Geometry: see drawing. Coordinates: mm, zero at the bounding-box minimum. Round coordinates to 2 decimals unless told otherwise and drop trailing zeros. Write each loop counter-clockwise with the first axis right and the second up, starting at its lowest first coordinate (ties: lowest second). Pieces come first, ordered by that corner, then holes. Notation, with made-up numbers: (-29, 24.25) - (28, 24.25) arc R18 cw to (28, 59.25) - close; hole circle Ø11 at (6.25, 38.25). An arc over 180 degrees is marked (long way). One line per item, written item: value. Start each with the question number.
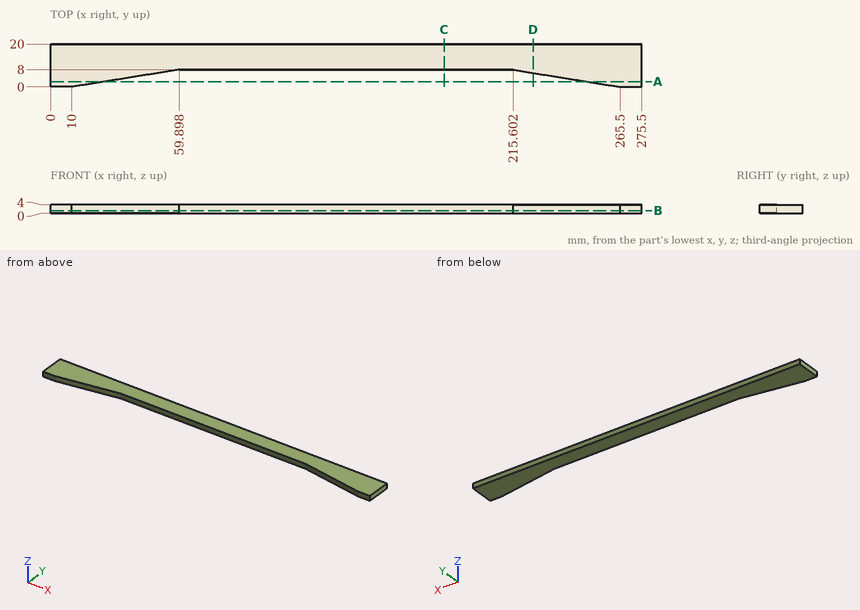
Q1. Cut plane B-B, the plane z = 1.35. Output: boundary loops of the cut face in (x, y), and give its area (4 significant figures).
Q2. Cut plane C-C, the plane x = 183.5. Output: boundary loops of the cut face in (y, z).
Q3. Material intervals for probe 1 along Y at (x, z) = (145.5, 0.4); probe 2 along Y at (x, z) = (241, 1.2), sorted ascending. Write a range as from..to.
Q4. Cut plane D-D, the plane x = 225. Output: boundary loops of the cut face in (y, z), and give its area (3 significant figures).
Q5. Cut plane A-A, the plane y = 2.5. Output: boundary loops of the cut face in (x, z).
A:
1. outline: (0, 0) - (10, 0) - (59.9, 8) - (215.6, 8) - (265.5, 0) - (275.5, 0) - (275.5, 20) - (0, 20) - close
1. area: 3,865 mm²
2. outline: (8, 0) - (20, 0) - (20, 4) - (8, 4) - close
3. probe 1: y = 8..20
3. probe 2: y = 3.93..20
4. outline: (6.49, 0) - (20, 0) - (20, 4) - (6.49, 4) - close
4. area: 54.0 mm²
5. outline: (0, 0) - (25.59, 0) - (25.59, 4) - (0, 4) - close; (249.91, 0) - (275.5, 0) - (275.5, 4) - (249.91, 4) - close
